Input: part model. Units: mm. Frame: model coordinates. Give positions to 0.01 mm unless a question says otherwise; leave off trailing zeros. Loops run counter-clockwise (first coordinate to the right, second up) from the corner with the lowest first, then second, coordinate; pieces in that order, holes last. Notation, with made-up numbers: (-9.75, 58.25) - (-2.75, 58.25) arc R15 cw to (-2.75, 83.25) - close; hole circle Ø6 at (2, 44.25). An arc over 180 degrees is marked (long way). Answer as a JSON object with one key per item and string values.
from build123d import *

# Parameters (mm, degrees)
F0_W     = 100
F0_H     = 314
F1_DEPTH = 18
F2_SIZE  = 17.99999
F3_R     = 17.99999


# Not quite as in the source:
# - a fillet or chamfer is up to 0.001 mm smaller than in the source, because OpenCascade refuses the exact size


with BuildPart() as f1:
    # F0 (on Front) → F1 (new body)
    with BuildSketch(Plane.XZ):
        Rectangle(F0_W, F0_H)
    extrude(amount=-F1_DEPTH)

    # F2 (size 18 in the source; OpenCascade refuses exactly that, so slightly less here)
    f2_edges = [f1.edges().sort_by_distance(p)[0] for p in [
        (-50, 0, 0),
    ]]
    chamfer(f2_edges, length=F2_SIZE)

    # F3 (radius 18 in the source; OpenCascade refuses exactly that, so slightly less here)
    f3_edges = [f1.edges().sort_by_distance(p)[0] for p in [
        (50, 0, 0),
    ]]
    fillet(f3_edges, radius=F3_R)


solid = f1.part
Item 1: Cut plane C-C (y = 14.5). Return loops of the section in (x, z), then the cut area to 3 significant figures.
Geometry check:
{"outline": "(-46.5, -157) - (49.66, -157) - (49.66, 157) - (-46.5, 157) - close", "area": "30,200 mm2"}
Item 2: Contact query for flat-ended pins moving along their axis: P1, Ø3, axis at y = 9, z = -124.5, coming from the -X side; P2, Ø8, axis at y = 6, z = -83.5, coming from the +X side; P3, Ø8, axis at y = 5.5, z = 72, coming from the -X side. Output: stop coordinate, or through.
Geometry check:
{"P1": "stops at x = -42.5", "P2": "stops at x = 48.12", "P3": "stops at x = -41.5"}
Item 3: Material intervals for line 1 (Y direction, x = -33, z = 14); line 2 (X direction, y = 2.75, z = 137); line 3 (X direction, y = 1.5, z = 108), sorted ascending. Write a range as [from, to].
Geometry check:
{"line 1": "y = [1, 18]", "line 2": "x = [-34.75, 41.56]", "line 3": "x = [-33.5, 39.19]"}
Item 4: Cut plane B-B (x = 37). Return loops of the section in (y, z).
Geometry check:
{"outline": "(0.71, -157) - (18, -157) - (18, 157) - (0.71, 157) - close"}
